The figure shows three views and two pictorial views of one solid part (mm, origin at its lowest corner). Answer the questions. Coordinates: 2 decimals unless noted, no trailing zeros. Write each loop counter-clockwise with the first axis right and the second up, starting at its lowest first coordinate (ties: lowest second). Pieces come first, ordered by that corner, then holes.
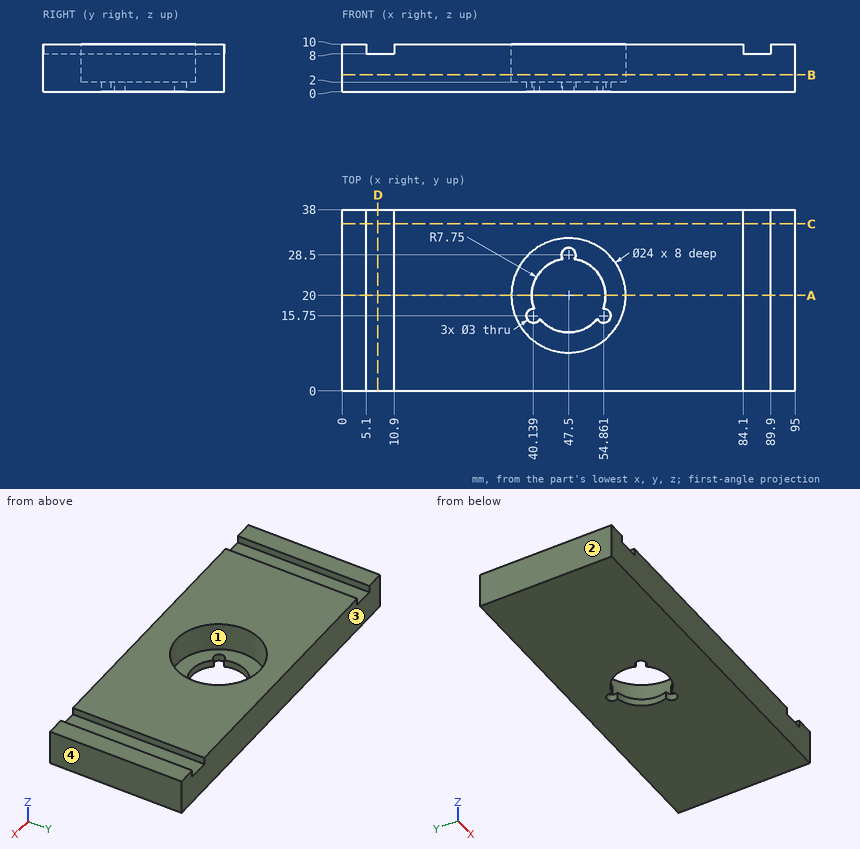
1. Flat-ended cylindrical pins translate along their axes: P1, Ø1.5, axis at x = 42, y = 13.5, coming from the +Z side; P2, Ø2.5, axis at x = 40.14, y = 15.75, coming from the -Z side. Find the tip coordinate at first contact, or state that the pin passes through.
Results found:
P1: stops at z = 2
P2: passes through
2. Section C-C on y = 35 is taken. Give the vertices of the cut face in (x, z), then the cut area to 3 significant figures.
Results found:
outline: (0, 0) - (95, 0) - (95, 10) - (89.9, 10) - (89.9, 8) - (84.1, 8) - (84.1, 10) - (10.9, 10) - (10.9, 8) - (5.1, 8) - (5.1, 10) - (0, 10) - close
area: 927 mm2
3. Section D-D on x = 7.5 is taken. Give the vertices of the cut face in (y, z).
Results found:
outline: (0, 0) - (38, 0) - (38, 8) - (0, 8) - close
4. Section A-A on y = 20 is taken. Give the vertices of the cut face in (x, z).
Results found:
outline: (0, 0) - (39.75, 0) - (39.75, 2) - (35.5, 2) - (35.5, 10) - (10.9, 10) - (10.9, 8) - (5.1, 8) - (5.1, 10) - (0, 10) - close; (55.25, 0) - (95, 0) - (95, 10) - (89.9, 10) - (89.9, 8) - (84.1, 8) - (84.1, 10) - (59.5, 10) - (59.5, 2) - (55.25, 2) - close
5. For a pull along X with two mould halves and no side action, classify the marked faces 1, 2, 3 and 4 as pulls with the +X half, pulls with the -X half, needs draft (parallel to the pull), parting line crosses it, or undercut.
Results found:
face 1: undercut
face 2: pulls with the -X half
face 3: needs draft
face 4: pulls with the +X half
6. Find the intervals of material crossed by L1, parallel to X at y = 28.5, z = 1.5; L2, parallel to Y at x = 47.5, z = 4.25; L3, parallel to X at y = 32.5, z = 8.5, in increasing order.
Results found:
L1: x = 0 to 46, 49 to 95
L2: y = 0 to 8, 32 to 38
L3: x = 0 to 5.1, 10.9 to 84.1, 89.9 to 95
7. Section B-B on z = 3.5 is taken. Give the vertices of the cut face in (x, y).
Results found:
outline: (0, 0) - (95, 0) - (95, 38) - (0, 38) - close; hole circle Ø24 at (47.5, 20)
